Verification items for the finished model (mm, model axes). Face numbers are marked on the shaded views. A direction names the side the tool comes from. Round coordinates to 2 decimals unless told otherwise and drop trailing zeros. Write each loop counter-clockwise with the first axis right and the second up, starting at its lowest first coordinate (ties: lowest second). Pieces come first, ordered by that corner, then holes. Notation, with made-up numbers: (-27, 45.5) - (-13, 45.5) arc R10 ccw to (-13, 64.5) - close; hole circle Ø7 at (23, -21). An arc over 180 degrees is marked (long way). Answer as a JSON object with one key per item and string values.
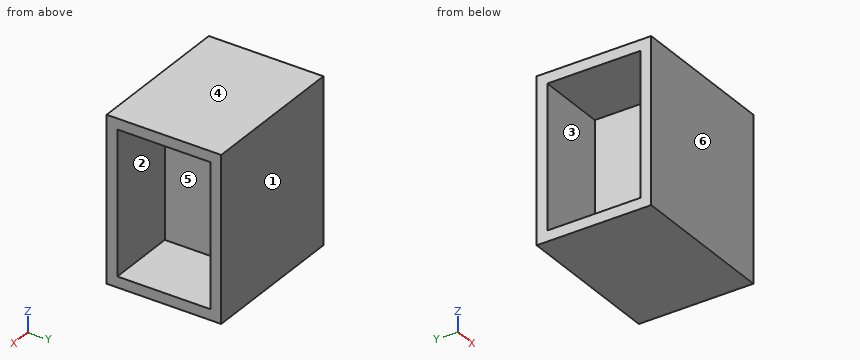
```python
from build123d import *

# Parameters (mm, degrees)
SKETCH1_W           = 42.4
SKETCH1_H           = 32.12
BOSS_EXTRUDE1_DEPTH = 3
BOSS_EXTRUDE2_DEPTH = 40
SKETCH3_W           = 42.4
SKETCH3_H           = 32.12
BOSS_EXTRUDE3_DEPTH = 3


with BuildPart() as part:
    # Sketch1 → Boss-Extrude1 (new body)
    with BuildSketch(Plane.XY):
        Rectangle(SKETCH1_W, SKETCH1_H)
    extrude(amount=BOSS_EXTRUDE1_DEPTH)

    # Sketch2 → Boss-Extrude2 (add)
    with BuildSketch(Plane.XY.offset(3)):
        Polygon((-21.2, 16.06), (-21.2, 13.06), (-1.5, 13.06), (-1.5, -13.06), (-21.2, -13.06), (-21.2, -16.06), (21.2, -16.06), (21.2, -13.06), (1.5, -13.06), (1.5, 13.06), (21.2, 13.06), (21.2, 16.06), align=None)
    extrude(amount=BOSS_EXTRUDE2_DEPTH)

    # Sketch3 → Boss-Extrude3 (add)
    with BuildSketch(Plane.XY.offset(43)):
        Rectangle(SKETCH3_W, SKETCH3_H)
    extrude(amount=BOSS_EXTRUDE3_DEPTH)


solid = part.part
```
1. Cross-section at A-A (x = 7.5). Record the boundary of the cut face in (y, z).
Completed:
{"outline": "(-16.06, 0) - (16.06, 0) - (16.06, 46) - (-16.06, 46) - close; hole (-13.06, 3) - (13.06, 3) - (13.06, 43) - (-13.06, 43) - close"}
2. Material ranges on probe 1 along Z at (x, y) = (9, 10); probe 2 along Y at (x, z) = (19, 29.5); probe 3 along X at (y, z) = (-3, 25.5), recorded low to high. Write a range as from..to.
Completed:
{"probe 1": "z = 0..3, 43..46", "probe 2": "y = -16.06..-13.06, 13.06..16.06", "probe 3": "x = -1.5..1.5"}
3. Go/stop test with flat-tipped pins: pin 1 (13 mm diameter, centred on y = -3.5, z = 13.5, fed in from +X); pin 2 (1.5 mm diameter, centred on x = 12.5, y = 0, fed in from -Z). Record where each tip stops, or that it passes through.
Completed:
{"pin 1": "stops at x = 1.5", "pin 2": "stops at z = 0"}
4. Cross-section at C-C (z = 11). Record the boundary of the cut face in (x, y), plus the area to 3 significant figures.
Completed:
{"outline": "(-21.2, -16.06) - (21.2, -16.06) - (21.2, -13.06) - (1.5, -13.06) - (1.5, 13.06) - (21.2, 13.06) - (21.2, 16.06) - (-21.2, 16.06) - (-21.2, 13.06) - (-1.5, 13.06) - (-1.5, -13.06) - (-21.2, -13.06) - close", "area": "333 mm^2"}
5. Cross-section at B-B (y = 0.5). Record the boundary of the cut face in (x, z).
Completed:
{"outline": "(-21.2, 0) - (21.2, 0) - (21.2, 3) - (1.5, 3) - (1.5, 43) - (21.2, 43) - (21.2, 46) - (-21.2, 46) - (-21.2, 43) - (-1.5, 43) - (-1.5, 3) - (-21.2, 3) - close"}
6. Mould release check, pull along Z, two halves, no side actions. Record for the marked faces 4, 5 and 6: released by +Z, released by -Z, zero draft, split by the parting line, or undercut.
Completed:
{"face 4": "released by +Z", "face 5": "undercut", "face 6": "zero draft"}
7. Access from +Z, -Z, +X, -X, +Y, -Y to the whole of each face (thin tool, end or side, straight path). Record for the marked faces 1, 2 and 3.
Completed:
{"face 1": "+Z, -Z, +X, -X, +Y", "face 2": "+X", "face 3": "-X"}
